```python
from build123d import *

# Parameters (mm, degrees)
F0_W      = 190
F0_H      = 25
F1_DEPTH  = 3
F3_D      = 18
F4_D      = 18
F5_W      = 12
F5_H      = 25
F6_DEPTH  = 23
F7_R      = 5
F9_D      = 7
F11_DEPTH = 50
F12_DEPTH = 25.4
F13_W     = 30
F13_H     = 7
F13_W_2   = 29.7052872181
F14_DEPTH = 70


with BuildPart() as f1:
    # F0 (on Front) → F1 (new body)
    with BuildSketch(Plane.XZ):
        with Locations((-95, 12.5)):
            Rectangle(F0_W, F0_H)
    extrude(amount=F1_DEPTH)

    # F3 (through all)
    with Locations(Plane.XZ.offset(3)):
        with Locations((-78.1028885841, 12.5)):
            Hole(F3_D / 2)

    # F4 (through all)
    with Locations(Plane.XZ.offset(3)):
        with Locations((-101.1028885841, 12.5)):
            Hole(F4_D / 2)

    # F5 (on face) → F6 (join)
    with BuildSketch(Plane(origin=(0, 0, 0), x_dir=(-1, 0, 0), z_dir=(0, 1, 0))):
        with Locations((171, 12.5)):
            Rectangle(F5_W, F5_H)
        with Locations((16, 12.5)):
            Rectangle(F5_W, F5_H)
    extrude(amount=F6_DEPTH)

    # F7
    f7_edges = [f1.edges().sort_by_distance(p)[0] for p in [
        (-10, 23, 12.5),
        (-22, 23, 12.5),
        (-165, 23, 12.5),
        (-177, 23, 12.5),
    ]]
    fillet(f7_edges, radius=F7_R)

    # F9 (through all)
    with Locations(Plane(origin=(0, 0, 0), x_dir=(1, 0, 0), z_dir=(0, 0, -1))):
        with Locations((-16, -17), (-171, -17)):
            Hole(F9_D / 2)

    # F10 (on face) → F11 (cut)
    with BuildSketch(Plane(origin=(0, 0, 0), x_dir=(1, 0, 0), z_dir=(0, 0, -1))):
        with BuildLine():
            Line((-10, 0), (-10, -8.7173189968))
            add(Edge.make_bspline(
                [(-10, -8.7173189968), (-7.7008124763, -8.7173189968), (-7.5862252656, -4.5655746788), (-7.4716380548, -0.4138303608), (-9.7594039535, 0)],
                knots=[0, 0, 0, 1.5209375403, 1.5209375403, 3.0418750806, 3.0418750806, 3.0418750806], degree=2, weights=[1, 0.7245129853, 1, 0.7245129853, 1]))
            Line((-9.7594039535, 0), (-10, 0))
        make_face()
        with BuildLine():
            add(Edge.make_bspline(
                [(-22.2405960465, 0), (-24.5283619452, -0.4138303608), (-24.4137747344, -4.5655746788), (-24.2991875237, -8.7173189968), (-22, -8.7173189968)],
                knots=[3.2413102266, 3.2413102266, 3.2413102266, 4.7622477669, 4.7622477669, 6.2831853072, 6.2831853072, 6.2831853072], degree=2, weights=[1, 0.7245129853, 1, 0.7245129853, 1]))
            Line((-22, -8.7173189968), (-22, 0))
            Line((-22, 0), (-22.2405960465, 0))
        make_face()
        with BuildLine():
            add(Edge.make_bspline(
                [(-165, -8.7173189968), (-162.7008124763, -8.7173189968), (-162.5862252656, -4.5655746788), (-162.4716380548, -0.4138303608), (-164.7594039535, 0)],
                knots=[0, 0, 0, 1.5209375403, 1.5209375403, 3.0418750806, 3.0418750806, 3.0418750806], degree=2, weights=[1, 0.7245129853, 1, 0.7245129853, 1]))
            Line((-164.7594039535, 0), (-165, 0))
            Line((-165, 0), (-165, -8.7173189968))
        make_face()
        with BuildLine():
            add(Edge.make_bspline(
                [(-177.2405960465, 0), (-179.5283619452, -0.4138303608), (-179.4137747344, -4.5655746788), (-179.2991875237, -8.7173189968), (-177, -8.7173189968)],
                knots=[3.2413102266, 3.2413102266, 3.2413102266, 4.7622477669, 4.7622477669, 6.2831853072, 6.2831853072, 6.2831853072], degree=2, weights=[1, 0.7245129853, 1, 0.7245129853, 1]))
            Line((-177, -8.7173189968), (-177, 0))
            Line((-177, 0), (-177.2405960465, 0))
        make_face()
    extrude(amount=-F11_DEPTH, mode=Mode.SUBTRACT)

    # F10 (on face) → F12 (cut)
    with BuildSketch(Plane(origin=(0, 0, 0), x_dir=(1, 0, 0), z_dir=(0, 0, -1))):
        with BuildLine():
            add(Edge.make_bspline(
                [(-22, -8.7173189968), (-17.8140176358, -8.7173189968), (-19.9070088179, -2.1630499978), (-22, 4.3912190013), (-24.0929911821, -2.1630499978), (-26.1859823642, -8.7173189968), (-22, -8.7173189968)],
                knots=[0, 0, 0, 2.0943951024, 2.0943951024, 4.1887902048, 4.1887902048, 6.2831853072, 6.2831853072, 6.2831853072], degree=2, weights=[1, 0.5, 1, 0.5, 1, 0.5, 1]))
        make_face()
        with BuildLine():
            add(Edge.make_bspline(
                [(-10, -8.7173189968), (-5.8140176358, -8.7173189968), (-7.9070088179, -2.1630499978), (-10, 4.3912190013), (-12.0929911821, -2.1630499978), (-14.1859823642, -8.7173189968), (-10, -8.7173189968)],
                knots=[0, 0, 0, 2.0943951024, 2.0943951024, 4.1887902048, 4.1887902048, 6.2831853072, 6.2831853072, 6.2831853072], degree=2, weights=[1, 0.5, 1, 0.5, 1, 0.5, 1]))
        make_face()
        with BuildLine():
            add(Edge.make_bspline(
                [(-177, -8.7173189968), (-172.8140176358, -8.7173189968), (-174.9070088179, -2.1630499978), (-177, 4.3912190013), (-179.0929911821, -2.1630499978), (-181.1859823642, -8.7173189968), (-177, -8.7173189968)],
                knots=[0, 0, 0, 2.0943951024, 2.0943951024, 4.1887902048, 4.1887902048, 6.2831853072, 6.2831853072, 6.2831853072], degree=2, weights=[1, 0.5, 1, 0.5, 1, 0.5, 1]))
        make_face()
        with BuildLine():
            add(Edge.make_bspline(
                [(-165, -8.7173189968), (-160.8140176358, -8.7173189968), (-162.9070088179, -2.1630499978), (-165, 4.3912190013), (-167.0929911821, -2.1630499978), (-169.1859823642, -8.7173189968), (-165, -8.7173189968)],
                knots=[0, 0, 0, 2.0943951024, 2.0943951024, 4.1887902048, 4.1887902048, 6.2831853072, 6.2831853072, 6.2831853072], degree=2, weights=[1, 0.5, 1, 0.5, 1, 0.5, 1]))
        make_face()
    extrude(amount=-F12_DEPTH, mode=Mode.SUBTRACT)

    # F13 (on face) → F14 (cut)
    with BuildSketch(Plane.XZ.offset(3)):
        with Locations((-15, 3.5)):
            Rectangle(F13_W, F13_H)
        with Locations((-175.147356391, 3.5)):
            Rectangle(F13_W_2, F13_H)
    extrude(amount=-F14_DEPTH, mode=Mode.SUBTRACT)


solid = f1.part
```
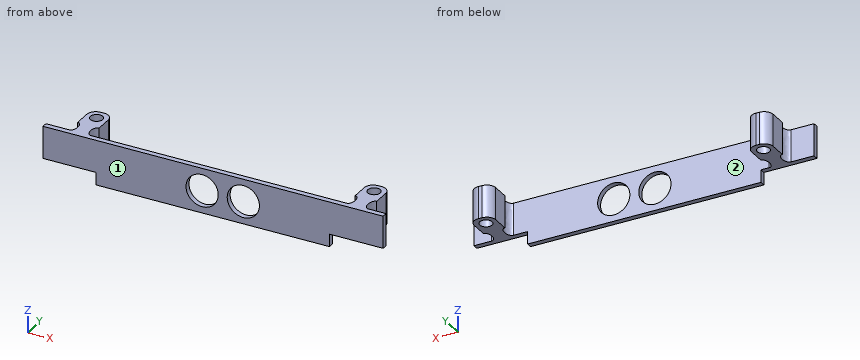
Input: part model. Units: mm. Frame: model coordinates. Face numbers are marked on the shaded views. Coordinates: 2 decimals unless noted, no trailing zeros. Order: outer loops, then holes, each group sorted by start corner. A loop starts at its lowest first (then second) coordinate and runs counter-clockwise, first axis right, second up. Notation, with made-up numbers: (-37.5, 76.25) - (-29.5, 76.25) arc R16 cw to (-29.5, 90.25) - close; hole circle Ø7 at (-39, 62). An arc over 180 degrees is marked (long way). Return JSON: item names as keys, results as strings.
Q1. Cut plane D-D (x = -73). Return loops of the section in (y, z), then the cut area to 3 significant figures.
The answers:
{"outline": "(-3, 0) - (0, 0) - (0, 5.09) - (-3, 5.09) - close; (-3, 19.91) - (0, 19.91) - (0, 25) - (-3, 25) - close", "area": "30.5 mm2"}
Q2. Cut plane A-A (x = -105). Return loops of the section in (y, z), then the cut area to 3 significant figures.
The answers:
{"outline": "(-3, 0) - (0, 0) - (0, 4.39) - (-3, 4.39) - close; (-3, 20.61) - (0, 20.61) - (0, 25) - (-3, 25) - close", "area": "26.3 mm2"}
Q3. First-contact query: pin 1 (10 mm diameter, centred on y = 15, z = 15.5, fed in from +X); pin 2 (10.5 mm diameter, centred on x = -5.5, z = 12, fed in from +Y); pin 3 (12.5 mm diameter, centred on x = -100, z = 16, fed in from +Y). Flat tips, straight axial feed; report the tip coordinate or a pass-through.
The answers:
{"pin 1": "stops at x = -10", "pin 2": "stops at y = 20.63", "pin 3": "stops at y = 0"}
Q4. Ray query, probe 1 along X at (y, z) = (16.5, 15); probe 2 along Y at (x, z) = (-16, 21); probe 3 along X at (y, z) = (17.75, 16.75). Return the intervals inside material, ascending.
The answers:
{"probe 1": "x = -177 to -174.46, -167.54 to -165, -22 to -19.46, -12.54 to -10", "probe 2": "y = -3 to 13.5, 20.5 to 23", "probe 3": "x = -177 to -174.42, -167.58 to -165, -22 to -19.42, -12.58 to -10"}
Q5. Cut plane B-B (z = 5.25). Return loops of the section in (x, y).
The answers:
{"outline": "(-160.29, -3) - (-106.44, -3) - (-106.44, 0) - (-160.29, 0) - close; (-95.77, -3) - (-83.44, -3) - (-83.44, 0) - (-95.77, 0) - close; (-72.77, -3) - (-30, -3) - (-30, 0) - (-72.77, 0) - close"}
Q6. Draft query along X for the marked faces 1 and 2. Return one class per face: +X half, -X half, draft (parallel to the pull), parting line (faces both ways), or undercut.
The answers:
{"face 1": "draft", "face 2": "undercut"}
Q7. Cut plane C-C (z = 12.5). State how many separate pieces and enclosed holes the cut face has, then the cut area to 3 significant figures.
The answers:
{"separate pieces": "3", "enclosed holes": "2", "area": "849 mm2"}
